Here's how the part is built. I have some questions about the finished solid (model axes, mm). Round coordinates to 2 decimals unless told otherwise and drop trailing zeros. Write each loop counter-clockwise with the first axis right and the second up, starting at its lowest first coordinate (ties: lowest second). Pieces come first, ordered by that corner, then holes. Notation, with made-up numbers: (23.5, -38.75) -> (68.5, -38.75) arc R31 ccw to (68.5, -2.75) -> close; hole circle Ø4 at (-18.75, -5.75). An arc over 180 degrees is marked (long way). Answer in a Markdown table with one row per item.
from build123d import *

# Parameters (mm, degrees)
BOSS_EXTRUDE1_DEPTH = 78
SKETCH2_W           = 8.5
SKETCH2_H           = 6
BOSS_EXTRUDE2_DEPTH = 8.5
SKETCH3_R           = 1.5
CUT_EXTRUDE1_DEPTH  = 100


with BuildPart() as part:
    # Sketch1 → Boss-Extrude1 (new body)
    with BuildSketch(Plane.XY):
        with BuildLine():
            Line((-4.25, -45.5), (4.25, -45.5))
            Line((4.25, -45.5), (4.25, -42.286966077))
            ThreePointArc((4.25, -42.286966077), (0, -42.5), (-4.25, -42.286966077))
            Line((-4.25, -42.286966077), (-4.25, -45.5))
        make_face()
    extrude(amount=BOSS_EXTRUDE1_DEPTH)

    # Sketch2 → Boss-Extrude2 (add)
    with BuildSketch(Plane(origin=(0, -42.5, 0), x_dir=(-1, 0, 0), z_dir=(0, -1, 0))):
        with Locations((0, -75)):
            Rectangle(SKETCH2_W, SKETCH2_H)
        with Locations((0, -3)):
            Rectangle(SKETCH2_W, SKETCH2_H)
    extrude(amount=-BOSS_EXTRUDE2_DEPTH)

    # Sketch3 → Cut-Extrude1 (cut)
    with BuildSketch(Plane(origin=(0, 0, 0), x_dir=(-1, 0, 0), z_dir=(0, 0, -1))):
        with Locations((0, -37)):
            Circle(SKETCH3_R)
    extrude(amount=-CUT_EXTRUDE1_DEPTH, mode=Mode.SUBTRACT)


solid = part.part
1) I need wall thicknesses on line 1 (Z direction, x = -0.75, y = -34.5); line 2 (Y direction, x = 0, z = 1.75); line 3 (Y direction, x = -0.5, z = 22). Which ranges of each line are inside material? Lowest first, please. Write a range as [from, to].
Response:
| item | result |
|---|---|
| line 1 | z = [0, 6], [72, 78] |
| line 2 | y = [-45.5, -38.5], [-35.5, -34] |
| line 3 | y = [-45.5, -42.5] |
2) I want a section at C-C, the plane x = -3.5. List the corners of the cut face in (y, z) for me, and give its area (3 significant figures).
Response:
| item | result |
|---|---|
| outline | (-45.5, 0) -> (-34, 0) -> (-34, 6) -> (-42.36, 6) -> (-42.36, 72) -> (-34, 72) -> (-34, 78) -> (-45.5, 78) -> close |
| area | 346 mm^2 |
3) I want a section at A-A, the plane y = -37. List the corners of the cut face in (x, z) for me, and give its area (3 significant figures).
Response:
| item | result |
|---|---|
| outline | (-4.25, 0) -> (-1.5, 0) -> (-1.5, 6) -> (-4.25, 6) -> close; (-4.25, 72) -> (-1.5, 72) -> (-1.5, 78) -> (-4.25, 78) -> close; (1.5, 0) -> (4.25, 0) -> (4.25, 6) -> (1.5, 6) -> close; (1.5, 72) -> (4.25, 72) -> (4.25, 78) -> (1.5, 78) -> close |
| area | 66.0 mm^2 |
4) We'd pull the mould along X, two halves only. Please class faces 1 (the face through (0, -34, 75)), 2 (the face through (-4.25, -44, 38)), 3 (the face through (0.1, -42.5, 38.5)): +X half, -X half, draft (parallel to the pull), parting line (faces both ways), or undercut.
Response:
| item | result |
|---|---|
| face 1 | draft |
| face 2 | -X half |
| face 3 | undercut |
5) I want a section at D-D, the plane z = 48.5. List the corners of the cut face in (x, y) for me, and give its area (3 significant figures).
Response:
| item | result |
|---|---|
| outline | (-4.25, -45.5) -> (4.25, -45.5) -> (4.25, -42.29) arc R42.5 cw to (-4.25, -42.29) -> close |
| area | 26.1 mm^2 |
6) I want a section at B-B, the plane x = 0. List the corners of the cut face in (y, z) for me, and give its area (3 significant figures).
Response:
| item | result |
|---|---|
| outline | (-45.5, 0) -> (-38.5, 0) -> (-38.5, 6) -> (-42.5, 6) -> (-42.5, 72) -> (-38.5, 72) -> (-38.5, 78) -> (-45.5, 78) -> close; (-35.5, 0) -> (-34, 0) -> (-34, 6) -> (-35.5, 6) -> close; (-35.5, 72) -> (-34, 72) -> (-34, 78) -> (-35.5, 78) -> close |
| area | 300 mm^2 |
